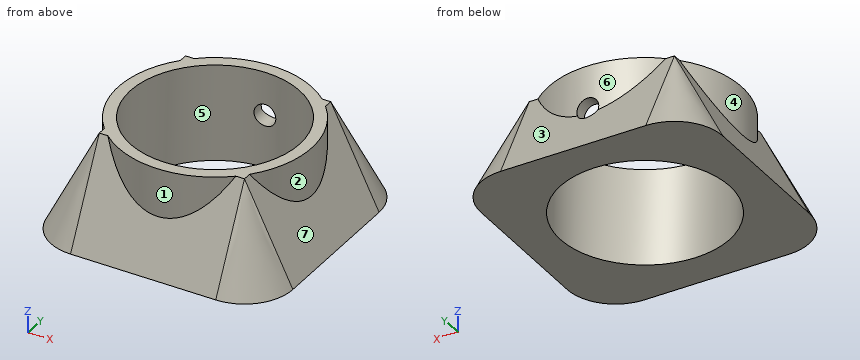
from build123d import *

# Parameters (mm, degrees)
F0_R         = 20
F1_DEPTH     = 20
F2_T1_DEPTH  = 30
F2_T3_DEPTH  = 30
F2_T6_ANGLE  = 90
F2_T8_ANGLE  = 90
F2_T10_ANGLE = 90
F2_T12_ANGLE = 90
F0_R_2       = 17.5
F3_DEPTH     = 20
F4_R         = 2.25
F5_DEPTH     = 25


# Not quite as in the source:
# - a fillet or chamfer that OpenCascade refuses, or shapes differently, is made with other operations: its cross-section is extruded or revolved along the edge and cut away or added


with BuildPart() as f1:
    # F0 (on Top) → F1 (new body)
    with BuildSketch(Plane.XY):
        with BuildLine():
            ThreePointArc((25, 15), (22.0710678119, 22.0710678119), (15, 25))
            Line((15, 25), (-15, 25))
            ThreePointArc((-15, 25), (-22.0710678119, 22.0710678119), (-25, 15))
            Line((-25, 15), (-25, -15))
            ThreePointArc((-25, -15), (-22.0710678119, -22.0710678119), (-15, -25))
            Line((-15, -25), (15, -25))
            ThreePointArc((15, -25), (22.0710678119, -22.0710678119), (25, -15))
            Line((25, -15), (25, 15))
        make_face()
        Circle(F0_R, mode=Mode.SUBTRACT)
    extrude(amount=F1_DEPTH)

    # F2: chamfer of 20 x 10 on 1 edges, made by hand

    # F2_s2 → F2_t1 (cut)
    with BuildSketch(Plane.YZ.offset(-15)):
        Polygon((-25, 0), (-15, 20), (-25, 20), align=None)
        Polygon((25, 0), (15, 20), (25, 20), align=None)
    extrude(amount=F2_T1_DEPTH, mode=Mode.SUBTRACT)

    # F2_s4 → F2_t3 (cut)
    with BuildSketch(Plane.XZ.offset(-15)):
        Polygon((25, 0), (15, 20), (25, 20), align=None)
        Polygon((-25, 0), (-15, 20), (-25, 20), align=None)
    extrude(amount=F2_T3_DEPTH, mode=Mode.SUBTRACT)

    # F2_s5 → F2_t6 (revolve, cut)
    with BuildSketch(Plane.XZ.offset(15)):
        Polygon((-25, 0), (-15, 20), (-25, 20), align=None)
    revolve(axis=Axis((-15, -15, 20), (0, 0, 1)), revolution_arc=F2_T6_ANGLE, mode=Mode.SUBTRACT)

    # F2_s7 → F2_t8 (revolve, cut)
    with BuildSketch(Plane.YZ.offset(15)):
        Polygon((-25, 0), (-15, 20), (-25, 20), align=None)
    revolve(axis=Axis((15, -15, 20), (0, 0, 1)), revolution_arc=F2_T8_ANGLE, mode=Mode.SUBTRACT)

    # F2_s9 → F2_t10 (revolve, cut)
    with BuildSketch(Plane.XZ.offset(-15)):
        Polygon((25, 0), (15, 20), (25, 20), align=None)
    revolve(axis=Axis((15, 15, 20), (0, 0, 1)), revolution_arc=F2_T10_ANGLE, mode=Mode.SUBTRACT)

    # F2_s11 → F2_t12 (revolve, cut)
    with BuildSketch(Plane.YZ.offset(-15)):
        Polygon((25, 0), (15, 20), (25, 20), align=None)
    revolve(axis=Axis((-15, 15, 20), (0, 0, 1)), revolution_arc=F2_T12_ANGLE, mode=Mode.SUBTRACT)

    # F0 (on Top) → F3 (join)
    with BuildSketch(Plane.XY):
        Circle(F0_R)
        Circle(F0_R_2, mode=Mode.SUBTRACT)
    extrude(amount=F3_DEPTH)

    # F4 (on Front) → F5 (cut)
    with BuildSketch(Plane.XZ):
        with Locations((0, 11)):
            Circle(F4_R)
    extrude(amount=-F5_DEPTH, mode=Mode.SUBTRACT)


solid = f1.part
Design review of the part built by this model. Coordinates are the model's own, in mm. Face numbers are marked on the shaded views. A direction names the side the tool comes from. Round coordinates to 2 decimals unless told otherwise and drop trailing zeros. Write each loop counter-clockwise with the first axis right and the second up, starting at its lowest first coordinate (ties: lowest second). Pieces come first, ordered by that corner, then holes. Notation, with made-up numbers: (-29, -38.75) -> (-20, -38.75) arc R8 ccw to (-20, -33.75) -> close; hole circle Ø8 at (55.5, 69.5). An arc over 180 degrees is marked (long way). One line per item, written item: value. Start each with the question number.
Q1. Add section D-D (x = 5). Give the boundary of the cut face in (y, z), then the cut area to 3 significant figures.
Q2. Insertion check: P1, Ø8, axis at x = -2.5, z = 7.5, coming from the +Y side; P2, Ø2, axis at x = -1.5, z = 9.5, coming from the +Y side; P3, Ø6, axis at y = 19, z = 2.5, coming from the -X side. Each pin has a flat end and moves straight along its axis. Give the tip position at first contact, or say it passes through.
Q3. To check wall thickness, follow probe 1 along Y at (x, z) = (0, 14.25); probe 2 along Z at (x, y) = (0, 18.3); probe 3 along X at (y, z) = (18.7, 11). State the ranges of each line that lie inside material, in increasing order.
Q4. The part is to be moulded in two halves that separate along X. For the marked faces 4, 5, 6 and 7, say which applies: pulls with the +X half, pulls with the -X half, needs draft (parallel to the pull), parting line crosses it, or undercut.
Q5. Tool access review of the marked faces 1, 2 and 3: name each direction out of +Z, -Z, +X, -X, +Y, -Y from which nothing blocks a thin tool from reaching the whole face with its end or side.
Q6. Add section C-C (z = 1.5). Give the boundary of the cut face in (x, y).
Q7. Add section B-B (y = 0). Give the boundary of the cut face in (x, z), then the cut area to 3 significant figures.
Q8. Add section A-A (x = -1.5). Give the boundary of the cut face in (y, z).
Response:
1. outline: (-25, 0) -> (-16.77, 0) -> (-16.77, 20) -> (-19.36, 20) -> (-19.36, 11.27) -> close; (16.77, 0) -> (25, 0) -> (19.36, 11.27) -> (19.36, 20) -> (16.77, 20) -> close
1. area: 167 mm^2
2. P1: stops at y = 23.25
2. P2: stops at y = 20.75
2. P3: stops at x = -24.72
3. probe 1: y = -20 to -17.5, 17.5 to 20
3. probe 2: z = 0 to 8.75, 13.25 to 20
3. probe 3: x = -17.56 to -2.25, 2.25 to 17.56
4. face 4: pulls with the -X half
4. face 5: undercut
4. face 6: parting line crosses it
4. face 7: pulls with the +X half
5. face 1: +Z, -Y
5. face 2: +Z, +X
5. face 3: +Z, +Y
6. outline: (-24.25, -15) arc R9.25 ccw to (-15, -24.25) -> (15, -24.25) arc R9.25 ccw to (24.25, -15) -> (24.25, 15) arc R9.25 ccw to (15, 24.25) -> (-15, 24.25) arc R9.25 ccw to (-24.25, 15) -> close; hole circle Ø35 at (0, 0)
7. outline: (-25, 0) -> (-17.5, 0) -> (-17.5, 20) -> (-20, 20) -> (-20, 10) -> close; (17.5, 0) -> (25, 0) -> (20, 10) -> (20, 20) -> (17.5, 20) -> close
7. area: 150 mm^2
8. outline: (-25, 0) -> (-17.44, 0) -> (-17.44, 20) -> (-19.94, 20) -> (-19.94, 10.11) -> close; (17.44, 0) -> (25, 0) -> (20.34, 9.32) -> (17.44, 9.32) -> close; (17.44, 12.68) -> (19.94, 12.68) -> (19.94, 20) -> (17.44, 20) -> close
